Verification items for the finished model (mm, model axes). Face numbers are marked on the shaded views. A direction names the side the tool comes from. Round coordinates to 2 decimals unless told otherwise and drop trailing zeros. Write each loop counter-clockwise with the first axis right and the second up, starting at its lowest first coordinate (ties: lowest second). Pieces come first, ordered by that corner, then holes. Notation, with made-up numbers: (5, 40.25) - (49, 40.25) arc R26 ccw to (49, 73.25) - close; hole circle Ø6 at (-4, 4.25). An arc over 180 degrees is marked (long way). Write each question's results on one line, items separated by ' | '.
```python
from build123d import *

# Parameters (mm, degrees)
SALIENTE_EXTRUIR1_DEPTH = 170
CROQUIS2_W              = 170
CROQUIS2_H              = 20.000000000000014
SALIENTE_EXTRUIR2_DEPTH = 3.7
VACIADO1_T              = -1


with BuildPart() as part:
    # Croquis1 → Saliente-Extruir1 (new body)
    with BuildSketch(Plane(origin=(0, 0, 0), x_dir=(0, 0, -1), z_dir=(1, 0, 0))):
        with BuildLine():
            Line((80, 0), (100, 0))
            Line((100, 0), (99.99999999999999, -83.7))
            ThreePointArc((99.99999999999999, -83.7), (70.71067811865474, -154.41067811865474), (1.125e-14, -183.7))
            ThreePointArc((1.125e-14, -183.7), (-70.71067811865473, -154.41067811865474), (-99.99999999999999, -83.70000000000002))
            Line((-99.99999999999999, -83.70000000000002), (-100, -1.225e-14))
            Line((-100, -1.225e-14), (-80, -9.8e-15))
            Line((-80, -9.8e-15), (-79.99999999999999, -83.70000000000002))
            ThreePointArc((-79.99999999999999, -83.70000000000002), (-56.568542494923804, -140.26854249492382), (-1.47e-14, -163.70000000000002))
            ThreePointArc((-1.47e-14, -163.70000000000002), (56.5685424949238, -140.26854249492382), (80, -83.70000000000002))
            Line((80, -83.70000000000002), (80, 0))
        make_face()
    extrude(amount=SALIENTE_EXTRUIR1_DEPTH)

    # Croquis2 → Saliente-Extruir2 (add)
    with BuildSketch(Plane(origin=(0, 0, 0), x_dir=(1, 0, 0), z_dir=(0, 1, 0))):
        with Locations((85, 90)):
            Rectangle(CROQUIS2_W, CROQUIS2_H)
        with Locations((85, -90)):
            Rectangle(CROQUIS2_W, CROQUIS2_H)
    extrude(amount=SALIENTE_EXTRUIR2_DEPTH)

    # Vaciado1
    vaciado1_openings = [part.faces().sort_by_distance(p)[0] for p in [
        (85, -183.7, 0),
        (85, -40, 100),
        (85, -40, -100),
    ]]
    offset(amount=VACIADO1_T, openings=vaciado1_openings, kind=Kind.INTERSECTION)


solid = part.part
```
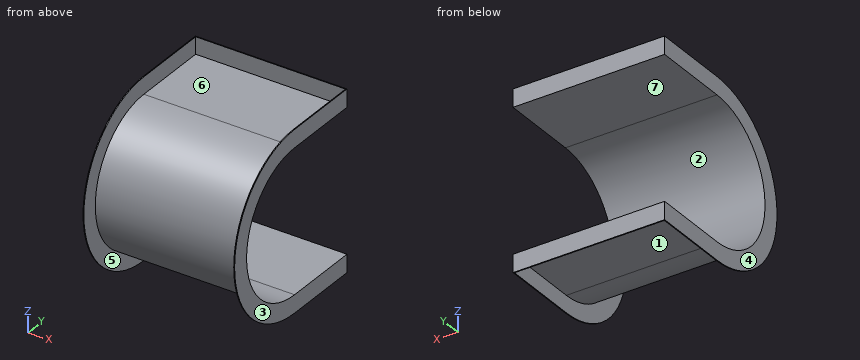
(1) Section check C-C (x = 55). Record the cut outline in (y, z), plus the area to 3 significant figures.
Answer:
outline: (-83.7, -81) - (2.7, -81) - (2.7, -100) - (3.7, -100) - (3.7, -80) - (-83.7, -80) arc R80 cw to (-83.7, 80) - (3.7, 80) - (3.7, 100) - (2.7, 100) - (2.7, 81) - (-83.7, 81) arc R81 ccw to start | area: 466 mm2
(2) Section check B-B (z = 0). Record the cut outline in (x, y).
Answer:
outline: (0, -183.7) - (1, -183.7) - (1, -164.7) - (169, -164.7) - (169, -183.7) - (170, -183.7) - (170, -163.7) - (0, -163.7) - close
(3) Thickness scan on L1, parallel to Z at x = 18.5, y = -8.5; L2, parallel to X at y = -62.5, z = -90; L3, parallel to Z at x = 58.5, y = -144. Record the ranges inside material, lowest first.
Answer:
L1: -81 to -80, 80 to 81 | L2: 0 to 1, 169 to 170 | L3: -54.08 to -52.57, 52.57 to 54.08
(4) Go/stop test with flat-tipped pins: pin 1 Ø4 at (x, y) = (127.5, -120.5) entering from +Z; pin 2 Ø4 at (x, y) = (123, -29) entering from -Z; pin 3 Ø12 at (x, y) = (25.5, -157.5) entering from -Z. Record where each tip stops, or that it passes through.
Answer:
pin 1: z = 73.14 | pin 2: z = -81 | pin 3: z = -44.32
(5) Section check D-D (z = 44). Record the cut outline in (x, y).
Answer:
outline: (0, -173.5) - (1, -173.5) - (1, -151.71) - (169, -151.71) - (169, -173.5) - (170, -173.5) - (170, -150.51) - (0, -150.51) - close
(6) Set-up check for the marked faces 4, 5, 6 and 7: record each of +Z, -Z, +X, -X, +Y, -Y from which the full face is reachable in a straight line by a thin tool's end or side.
Answer:
face 4: +Z, -Z, -X, +Y, -Y | face 5: -Y | face 6: +Z, -Y | face 7: +X, -X, +Y
(7) Section check A-A (y = -80.5). Record the cut outline in (x, z), plus the area to 3 significant figures.
Answer:
outline: (0, -100) - (1, -100) - (1, -81) - (169, -81) - (169, -100) - (170, -100) - (170, -80) - (0, -80) - close; (0, 80) - (170, 80) - (170, 100) - (169, 100) - (169, 81) - (1, 81) - (1, 100) - (0, 100) - close | area: 416 mm2
(8) Mould release check, pull along Z, two halves, no side actions. Record for the marked faces 1, 2 and 3: released by +Z, released by -Z, zero draft, split by the parting line, or undercut.
Answer:
face 1: released by -Z | face 2: undercut | face 3: zero draft
